Part model, mm, in its own coordinate system. A direction names the side the tool comes from. Coordinates: 2 decimals unless noted, no trailing zeros. Loops run counter-clockwise (first coordinate to the right, second up) from the corner with the lowest first, then second, coordinate; pieces in that order, holes last. Notation, with made-up numbers: M 3.5,46 L 21.5,46 A13 ccw 21.5,63 Z; hole C -35,13.25 d7. An arc over 180 degrees is marked long. Use a Markdown table: item, result. Add a question column.
1) Band-saw the part on A-A (y = 114). List the corners of the cut face in (x, z).
2) Band-saw the part on C-C (x = 157.5). List the corners of the cut face in (y, z).
3) Tool access for faces 4 (the flat face through (196.97, 146.89, 3.45)), 5 (the flat face through (157, 136, 7)), 6 (the flat face through (135.34, 114.51, 3.45)): list every direction of +Z, -Z, +X, -X, +Y, -Y with a clear straight run to the whole face (end or side of a thin tool).
4) Band-saw the part on B-B (z = 2). List the corners of the cut face in (x, y).
5) Band-saw the part on D-D (y = 120). List the corners of the cut face in (x, z), plus the area to 3 significant figures.
6) Wall check: probe 1 along Y at (x, z) = (179.5, 5.5); probe 2 along X at (y, z) = (136, 3); probe 3 along X at (y, z) = (150, 4.75). Give the ranges that are in metal, low to high. Write a range as from..to.
7) Pull direction Y, two halves, no side cores. Call faces 1 (the flat face through (174.396, 145.468, 3.542)), 2 (the flat face through (159, 135, 0)), 3 (the cylindrical face through (90.308, 118.538, 3.451)): released by +Y, released by -Y, zero draft, split by the parting line, or undercut.
8) Pin check, flat tips, straight feed: pin 1 Ø2 at (y, z) = (135.5, 1.5) entering from -X; pin 2 Ø2 at (y, z) = (160.5, 3) entering from +X; pin 3 Ø3 at (y, z) = (123.5, 3) entering from +X. Stop position of each tip, or through.
from build123d import *

# Parameters (mm, degrees)
PAD002_DEPTH             = 7
SKETCH025_R              = 3
POCKET018_DEPTH          = 15
POCKET019_DEPTH          = 98.908358
SKETCH028_R              = 3
POCKET021_DEPTH          = 7.001
CLONE002_PLACEMENT_ANGLE = 45


with BuildPart() as part:
    # Sketch023 → Pad002 (new body)
    with BuildSketch(Plane.XY):
        with BuildLine():
            Line((75.261973, 88.907358), (50.261973, 88.907358))
            Line((50.261973, 84.907358), (50.261973, 88.907358))
            Line((50.261973, 84.907358), (20.261973, 84.907358))
            Line((-9.396926, 3.420201), (20.261973, 84.907358))
            ThreePointArc((-9.396926, 3.420201), (-4.942745, -8.693059), (7.744606, -6.326221))
            Line((7.744606, -6.326221), (52.028155, 47.886022))
            ThreePointArc((75.261973, 58.907358), (62.404289, 56.012339), (52.028155, 47.886022))
            Line((75.261973, 88.907358), (75.261973, 58.907358))
        make_face()
    extrude(amount=PAD002_DEPTH)

    # Sketch025 (on Face4 of Pad002) → Pocket018 (cut)
    with BuildSketch(Plane(origin=(0, 84.907358, 0), x_dir=(-1, 0, 0), z_dir=(0, 1, 0))):
        with Locations((-35.261973, 3.5)):
            Circle(SKETCH025_R)
    extrude(amount=-POCKET018_DEPTH, mode=Mode.SUBTRACT)

    # Sketch026 (on Face2 of Pocket018) → Pocket019 (cut, through all)
    with BuildSketch(Plane(origin=(0, 88.907358, 0), x_dir=(-1, 0, 0), z_dir=(0, 1, 0))):
        Polygon((-75.261973, 7), (-75.261973, 0), (-71.220521, 7), align=None)
    extrude(amount=-POCKET019_DEPTH, mode=Mode.SUBTRACT)

    # Sketch028 → Pocket021 (cut, through all)
    with BuildSketch(Plane.XY.offset(7)):
        with Locations((54.303425, 73.770624)):
            Circle(SKETCH028_R)
    extrude(amount=-POCKET021_DEPTH, mode=Mode.SUBTRACT)


with BuildPart() as part_1:
    # Body002 placement: moved
    add(part.part.moved(Location((-250, 0, 0))))


with BuildPart() as part_2:
    # Clone002 placement: moved
    add(part_1.part.moved(Location((276.776695, -55.776695, 0))).rotate(Axis((276.776695, -55.776695, 0), (0, 0, -1)), CLONE002_PLACEMENT_ANGLE))


solid = part_2.part
Entries:
| question | item | result |
|---|---|---|
| 1 | outline | M 92.86,0 L 130.26,0 L 130.26,7 L 92.86,7 Z; M 189.01,0 L 199.44,0 L 193.72,7 L 189.01,7 Z |
| 2 | outline | M 116.75,0 L 158.85,0 L 158.85,7 L 116.75,7 Z |
| 3 | face 4 | +Z, -Z, +Y |
| 3 | face 5 | +Z, +X, -X, +Y, -Y |
| 3 | face 6 | +Z, -Z, -Y |
| 4 | outline | M 95.77,130.06 A10 ccw 101,111.05 L 170.65,118.07 A30 cw 194.04,110.24 L 215.27,131.47 L 198.41,148.33 L 195.58,145.5 L 186.81,154.27 L 176.2,143.66 L 172.53,147.34 L 183.14,157.94 L 174.37,166.71 Z; hole C 190.56,134.77 d6 |
| 5 | outline | M 90.05,0 L 205.44,0 L 199.72,7 L 90.05,7 Z |
| 5 | area | 788 mm2 |
| 6 | probe 1 | 117.65..147.47, 153.79..161.58 |
| 6 | probe 2 | 108.51..187.83, 193.3..210.73 |
| 6 | probe 3 | 138.53..175.01, 182.72..191.08 |
| 7 | face 1 | undercut |
| 7 | face 2 | zero draft |
| 7 | face 3 | split by the parting line |
| 8 | pin 1 | x = 105.29 |
| 8 | pin 2 | x = 181.58 |
| 8 | pin 3 | x = 208.42 |
